```python
from build123d import *

# Parameters (mm, degrees)
F1_DEPTH = 16.51
F2_R     = 7.62
F3_R     = 7.62
F4_R     = 5.08
F5_R     = 5.08
F6_SCALE = 0.75


with BuildPart() as f1:
    # F0 (on Front) → F1 (new body)
    with BuildSketch(Plane.XZ):
        Polygon((-13.8489005984, 31.7138343761), (-15.3638953721, 0), (15.0566186512, 0), (13.5416238775, 31.7138343761), align=None)
    extrude(amount=F1_DEPTH)

    # F2
    f2_edges = [f1.edges().sort_by_distance(p)[0] for p in [
        (-14.606398, -16.51, 15.856917),
    ]]
    fillet(f2_edges, radius=F2_R)

    # F3
    f3_edges = [f1.edges().sort_by_distance(p)[0] for p in [
        (14.299121, -16.51, 15.856917),
        (14.299121, 0, 15.856917),
        (-14.606398, 0, 15.856917),
    ]]
    fillet(f3_edges, radius=F3_R)

    # F4
    f4_edges = [f1.edges().sort_by_distance(p)[0] for p in [
        (-0.153638, 0, 0),
    ]]
    fillet(f4_edges, radius=F4_R)

    # F5
    f5_edges = [f1.edges().sort_by_distance(p)[0] for p in [
        (-0.153638, -16.51, 31.713834),
    ]]
    fillet(f5_edges, radius=F5_R)


with BuildPart() as f1_1:
    # F6: moved
    add(f1.part.scale(F6_SCALE))


solid = f1_1.part
```
The listing builds one solid part. Answer for the finished solid, in the listing's coordinates (mm). Round coordinates to 2 decimals unless told otherwise and drop trailing zeros. Loops run counter-clockwise (first coordinate to the right, second up) from the corner with the lowest first, then second, coordinate; pieces in that order, holes last. Notation, with made-up numbers: (57, 15.25) - (72, 15.25) arc R13 cw to (72, 39.25) - close; hole circle Ø9 at (55.25, -33). An arc over 180 degrees is marked (long way). Return JSON: item names as keys, results as strings. Group by question number.
1. The part is cut by section A-A on x = 1.5. Determine the outline of the cut face in (y, z), then the cut area to 3 significant figures.
2. Consider probe 1 along X at (y, z) = (-2.25, 15.5); probe 2 along Y at (x, z) = (4.5, 21.25); probe 3 along Y at (x, z) = (-9.25, 9.75). Determine where each line is inside the solid, lowest interval first.
3. Each of these flat-tipped pins is pushed along its axis until it touches: P1, Ø6, axis at y = -9, z = 11, coming from the +X side; P2, Ø1, axis at x = -8.5, y = -11, coming from the +Z side; P3, Ø3, axis at x = -7, z = 17.5, coming from the +Y side. Where does it stop, or does it pass through?
Resolved:
{
 "1": {"outline": "(-12.38, 3.81) arc R3.81 ccw to (-8.57, 0) - (-3.81, 0) arc R3.81 ccw to (0, 3.81) - (0, 19.98) arc R3.81 ccw to (-3.81, 23.79) - (-8.57, 23.79) arc R3.81 ccw to (-12.38, 19.98) - close", "area": "282 mm²"},
 "2": {"probe 1": "x = -9.61 to 9.38", "probe 2": "y = -12.16 to -0.22", "probe 3": "y = -10.84 to -1.55"},
 "3": {"P1": "stops at x = 10.86", "P2": "stops at z = 21.95", "P3": "stops at y = -0.02"}
}
